The model under review builds one solid part; all positions refer to its coordinate system, in mm. A direction names the side the tool comes from. Coordinates: 2 decimals unless noted, no trailing zeros. Order: outer loops, then holes, each group sorted by start corner. A loop starts at its lowest first (then second) coordinate and runs counter-clockwise, first axis right, second up. Notation, with made-up numbers: (-21, -17.75) - (31, -17.75) arc R29 ccw to (31, 11.25) - close; hole circle Ø8 at (-5.75, -12). An arc over 180 degrees is marked (long way). Answer in a Markdown table with one row per item.
```python
from build123d import *

# Parameters (mm, degrees)
EXTRUDE_1_DEPTH     = 1.5
EXTRUDE_2_DEPTH     = 10
SKETCH_3_R          = 1.75
CUT_EXTRUDE_1_DEPTH = 58.467382053
CUT_EXTRUDE_2_DEPTH = 80.907759323
EXTRUDE_3_DEPTH     = 1.2
EXTRUDE_4_DEPTH     = 1.2
SKETCH_7_R          = 1.75
EXTRUDE_5_DEPTH     = 1.2
EXTRUDE_START       = 1.2
SKETCH_8_R          = 1.75
EXTRUDE_6_DEPTH     = 1.2
SKETCH_9_W          = 24
SKETCH_9_H          = 10
CUT_EXTRUDE_4_DEPTH = 58.467382053


with BuildPart() as part:
    # 草图1 → 凸台-拉伸1 (new body)
    with BuildSketch(Plane.XY):
        Polygon((29.5, 6), (37.5, 0), (-37.5, 0), (-29.5, 6), (-29.5, 36), (-37.5, 42), (37.5, 42), (29.5, 36), align=None)
    extrude(amount=EXTRUDE_1_DEPTH)

    # 草图2 → 凸台-拉伸2 (add)
    with BuildSketch(Plane.XY.offset(1.5)):
        Polygon((29.5, 36), (37.5, 42), (-37.5, 42), (-29.5, 36), (-29.5, 6), (-37.5, 0), (37.5, 0), (29.5, 6), align=None)
        Polygon((28.3, 36.6), (33.9, 40.8), (-33.9, 40.8), (-28.3, 36.6), (-28.3, 5.4), (-33.9, 1.2), (33.9, 1.2), (28.3, 5.4), align=None, mode=Mode.SUBTRACT)
    extrude(amount=EXTRUDE_2_DEPTH)

    # 草图3 → 切除-拉伸1 (cut, through all)
    with BuildSketch(Plane(origin=(0, 42, 0), x_dir=(1, 0, 0), z_dir=(0, 1, 0))):
        with Locations(Location((-29.5, -6.5, 0), (0, 0, 270))):
            Circle(SKETCH_3_R)
        with Locations(Location((29.5, -6.5, 0), (0, 0, 180))):
            Circle(SKETCH_3_R)
    extrude(amount=-CUT_EXTRUDE_1_DEPTH, mode=Mode.SUBTRACT)

    # 草图4 → 切除-拉伸2 (cut, through all)
    with BuildSketch(Plane(origin=(29.5, 0, 0), x_dir=(0, 0, -1), z_dir=(1, 0, 0))):
        with BuildLine():
            Line((-2.466181259, 22.5318851), (-11.5, 36))
            Line((-11.5, 36), (-11.5, 6))
            Line((-11.5, 6), (-2.466181259, 19.4681149))
            ThreePointArc((-2.466181259, 19.4681149), (-2, 21), (-2.466181259, 22.5318851))
        make_face()
    extrude(amount=-CUT_EXTRUDE_2_DEPTH, mode=Mode.SUBTRACT)

    # 草图5 → 凸台-拉伸3 (add)
    with BuildSketch(Plane(origin=(29.5, 0, 0), x_dir=(0, 0, -1), z_dir=(1, 0, 0))):
        Polygon((-4.75, 25.936727957), (-8.25, 31.154720868), (-8.25, 36), (-4.75, 36), align=None)
        Polygon((-4.75, 16.063272043), (-8.25, 10.845279132), (-8.25, 6), (-4.75, 6), align=None)
    extrude(amount=-EXTRUDE_3_DEPTH)

    # 草图6 → 凸台-拉伸4 (add)
    with BuildSketch(Plane.ZY.offset(29.5)):
        Polygon((8.25, 6), (4.75, 6), (4.75, 16.063272043), (8.25, 10.845279132), align=None)
        Polygon((4.75, 25.936727957), (8.25, 31.154720868), (8.25, 36), (4.75, 36), align=None)
    extrude(amount=-EXTRUDE_4_DEPTH)

    # 草图7 → 凸台-拉伸5 (add)
    with BuildSketch(Plane.ZY.offset(29.5)):
        Polygon((9.5, 21), (9.5, 33.018289765), (8.061339847, 33.018289765), (0, 21), (8.061339847, 8.981710235), (9.5, 8.981710235), align=None)
        with Locations((6.5, 21)):
            Circle(SKETCH_7_R, mode=Mode.SUBTRACT)
    extrude(amount=EXTRUDE_5_DEPTH)

    # 草图8 → 凸台-拉伸6 (add)
    with BuildSketch(Plane(origin=(29.5, 0, 0), x_dir=(0, 0, -1), z_dir=(1, 0, 0)).offset(EXTRUDE_START)):
        Polygon((-9.5, 8.981710235), (-9.5, 33.018289765), (-8.061339847, 33.018289765), (0, 21), (-8.061339847, 8.981710235), align=None)
        with Locations(Location((-6.5, 21, 0), (0, 0, 180))):
            Circle(SKETCH_8_R, mode=Mode.SUBTRACT)
    extrude(amount=-EXTRUDE_6_DEPTH)

    # 草图9 → 切除-拉伸4 (cut, through all)
    with BuildSketch(Plane(origin=(0, 0, 0), x_dir=(-1, 0, 0), z_dir=(0, 0, -1))):
        with Locations((-12.5, 32)):
            Rectangle(SKETCH_9_W, SKETCH_9_H)
    extrude(amount=-CUT_EXTRUDE_4_DEPTH, mode=Mode.SUBTRACT)


solid = part.part
```
Item 1: We need section D-D, the plane y = 7. Write out the cut boundary in (x, z), then the cut area to 3 significant figures.
Check values:
| item | result |
|---|---|
| outline | (-29.5, 0) - (29.5, 0) - (29.5, 10.83) - (28.3, 10.83) - (28.3, 1.5) - (-28.3, 1.5) - (-28.3, 10.83) - (-29.5, 10.83) - close |
| area | 111 mm^2 |
Item 2: Tool access review of faces 4 (the face through (31.25, 4.23, 6.56)), 5 (the face through (-28.3, 25, 3)), 6 (the face through (-33.444, 3.042, 5.67)), 7 (the face through (30.108, 27.093, 4.087)): name each direction out of +Z, -Z, +X, -X, +Y, -Y from which nothing blocks a thin tool from reaching the whole face with its end or side.
Check values:
| item | result |
|---|---|
| face 4 | -Y |
| face 5 | +Z |
| face 6 | +Z, -Z, -X |
| face 7 | -Z, +X |
Item 3: To check wall thickness, follow line 1 (Y direction, x = 22.5, z = 6); line 2 (Y direction, x = 33, z = 9.5) (3 decimals); line 3 (Y direction, x = 33.5, z = 8). State the ranges of each line that lie inside material, in increasing order. Write a range as from..to.
Check values:
| item | result |
|---|---|
| line 1 | 0..1.2, 40.8..42 |
| line 2 | 0..1.2, 1.875..3.375, 38.625..40.125, 40.8..42 |
| line 3 | 0..1.2, 1.5..3, 39..40.5, 40.8..42 |
Item 4: Mouldability with a two-part tool opening along X and no side actions: class faces 1 (the face through (33.556, 2.958, 5.67)), 2 (the face through (-29.5, 32, 5)), 3 (the face through (0, 1.2, 6)) as +X half, -X half, draft (parallel to the pull), parting line (faces both ways), or undercut.
Check values:
| item | result |
|---|---|
| face 1 | +X half |
| face 2 | -X half |
| face 3 | undercut |
Item 5: We need section C-C, the plane x = -8. Write out the cut boundary in (y, z).
Check values:
| item | result |
|---|---|
| outline | (0, 0) - (42, 0) - (42, 11.5) - (40.8, 11.5) - (40.8, 1.5) - (1.2, 1.5) - (1.2, 11.5) - (0, 11.5) - close |
Item 6: We need section A-A, the plane y = 28. Write out the cut boundary in (x, z).
Check values:
| item | result |
|---|---|
| outline | (-30.7, 4.7) - (-29.5, 4.7) - (-29.5, 0) - (0.5, 0) - (0.5, 1.5) - (-28.3, 1.5) - (-28.3, 6.13) - (-29.5, 6.13) - (-29.5, 9.5) - (-30.7, 9.5) - close; (24.5, 0) - (29.5, 0) - (29.5, 4.7) - (30.7, 4.7) - (30.7, 9.5) - (29.5, 9.5) - (29.5, 6.13) - (28.3, 6.13) - (28.3, 1.5) - (24.5, 1.5) - close |
Item 7: Clearance check with flat-ended pins moving along their axes: pin 1 Ø0.6 at (x, z) = (28.5, 6) entering from -Y; pin 2 Ø2 at (x, z) = (-29.5, 6.5) entering from +Y; pin 3 Ø4 at (y, z) = (27, 1.5) entering from +X. State where each tip first meets the part, or that it passes through.
Check values:
| item | result |
|---|---|
| pin 1 | y = 6 |
| pin 2 | y = 36 |
| pin 3 | x = 29.5 |
